from build123d import *

# Parameters (mm, degrees)
CROQUIS1_RX                  = 19.25
CROQUIS1_RY                  = 16.2
CROQUIS1_RX_2                = 16.25
CROQUIS1_RY_2                = 13.2
SALIENTE_EXTRUIR1_DEPTH      = 33
CORTAR_EXTRUIR1_DEPTH        = 33
SALIENTE_EXTRUIR2_DEPTH      = 30
SALIENTE_EXTRUIR2_DEPTH_BACK = 30
CROQUIS4_W                   = 5.818790363
CROQUIS4_H                   = 5
CORTAR_EXTRUIR2_DEPTH        = 36
SALIENTE_EXTRUIR4_DEPTH      = 33
SALIENTE_EXTRUIR5_DEPTH      = 50
CORTAR_EXTRUIR3_DEPTH        = 50
CORTAR_EXTRUIR4_START        = -17.5
CORTAR_EXTRUIR4_DEPTH        = 17.5
CORTAR_EXTRUIR5_START        = -17.5
CORTAR_EXTRUIR5_DEPTH        = 17.5
CROQUIS11_R                  = 4.25
CORTAR_EXTRUIR6_DEPTH        = 4


with BuildPart() as part:
    # Croquis1 → Saliente-Extruir1 (new body)
    with BuildSketch(Plane(origin=(0, 0, 0), x_dir=(1, 0, 0), z_dir=(0, 1, 0))):
        with Locations(Location((0, 0), (0, 0, -90))):
            Ellipse(CROQUIS1_RX, CROQUIS1_RY)
        with Locations(Location((0, 0), (0, 0, -90))):
            Ellipse(CROQUIS1_RX_2, CROQUIS1_RY_2, mode=Mode.SUBTRACT)
    extrude(amount=SALIENTE_EXTRUIR1_DEPTH)

    # Croquis2 → Cortar-Extruir1 (cut)
    with BuildSketch(Plane(origin=(0, 33, 0), x_dir=(1, 0, 0), z_dir=(0, 1, 0))):
        Polygon((0, 0), (-7.647156017, 13.245262755), (-17.669144049, 13.245262755), (-24.728519105, -10.297452091), (-13.467362336, -13.245262755), (-7.647156017, -13.245262755), align=None)
    extrude(amount=-CORTAR_EXTRUIR1_DEPTH, mode=Mode.SUBTRACT)



with BuildPart() as body_2:
    # Croquis3 → Saliente-Extruir2 (new, two sides: drawn at the far end of the back side and taken through both)
    with BuildSketch(Plane.XY.offset(-SALIENTE_EXTRUIR2_DEPTH_BACK)):
        Polygon((16.2, 0), (22.018790363, 33), (16.2, 33), align=None)
    extrude(amount=SALIENTE_EXTRUIR2_DEPTH + SALIENTE_EXTRUIR2_DEPTH_BACK)

    # Croquis4 → Cortar-Extruir2 (cut)
    with BuildSketch(Plane(origin=(0, 33, 0), x_dir=(1, 0, 0), z_dir=(0, 1, 0))):
        with Locations((19.109395181, 27.5)):
            Rectangle(CROQUIS4_W, CROQUIS4_H)
        with Locations((19.109395181, -27.5)):
            Rectangle(CROQUIS4_W, CROQUIS4_H)
    extrude(amount=-CORTAR_EXTRUIR2_DEPTH, mode=Mode.SUBTRACT)


with BuildPart() as part_1:
    add(part.part)

    add(body_2.part)  # Saliente-Extruir4 merges body 2
    # Croquis5 → Saliente-Extruir4 (add)
    with BuildSketch(Plane(origin=(0, 33, 0), x_dir=(1, 0, 0), z_dir=(0, 1, 0))):
        Polygon((17.818457755, 0), (17.818457755, 7.5), (13.626292681, 7.5), (13.626292681, -7.5), (17.818457755, -7.5), align=None)
    extrude(amount=-SALIENTE_EXTRUIR4_DEPTH)

    # Croquis6 → Saliente-Extruir5 (add)
    with BuildSketch(Plane(origin=(0, 0, -25), x_dir=(-1, 0, 0), z_dir=(0, 0, -1))):
        Polygon((-22.018790363, 33), (-16.2, 0), (-19.345508023, -0.554637933), (-25.072873954, 31.926868346), (-25.262096019, 33), align=None)
    extrude(amount=-SALIENTE_EXTRUIR5_DEPTH)

    # Croquis7 → Cortar-Extruir3 (cut)
    with BuildSketch(Plane.XY.offset(25)):
        Polygon((16.2, 0), (19.443305655, 0), (19.345508023, -0.554637933), align=None)
    extrude(amount=-CORTAR_EXTRUIR3_DEPTH, mode=Mode.SUBTRACT)

    # Croquis8 → Cortar-Extruir4 (cut)
    with BuildSketch(Plane.XY.offset(25).offset(CORTAR_EXTRUIR4_START)):
        Polygon((16.2, 0), (22.018790363, 33), (16.2, 33), align=None)
    extrude(amount=CORTAR_EXTRUIR4_DEPTH, mode=Mode.SUBTRACT)

    # Croquis9 → Cortar-Extruir5 (cut)
    with BuildSketch(Plane(origin=(0, 0, -25), x_dir=(-1, 0, 0), z_dir=(0, 0, -1)).offset(CORTAR_EXTRUIR5_START)):
        Polygon((-16.2, 0), (-22.018790363, 33), (-16.2, 33), align=None)
    extrude(amount=CORTAR_EXTRUIR5_DEPTH, mode=Mode.SUBTRACT)

    # Croquis11 → Cortar-Extruir6 (cut)
    with BuildSketch(Plane(origin=(18.857018252, -3.325001094, 0), x_dir=(0, 0, -1), z_dir=(0.984807753012208, -0.17364817766693103, 0))):
        with Locations(Location((-15, 20.130372787, 0), (0, 0, 90))):
            Circle(CROQUIS11_R)
        with Locations(Location((15, 20.130372787, 0), (0, 0, 90))):
            Circle(CROQUIS11_R)
    extrude(amount=-CORTAR_EXTRUIR6_DEPTH, mode=Mode.SUBTRACT)


solid = part_1.part
For this review, take the finished solid that the model builds, in its own axes (mm). A direction names the side the tool comes from. Round coordinates to 2 decimals unless told otherwise and drop trailing zeros. Use one line per item in the form item = value.
Item 1: Tool access review of faces 1 (the flat face through (18.42, 12.6, -16.13)), 2 (the cylindrical face through (20.64, 15.87, -19.15)), 3 (the flat face through (-10, 17, 13.245)), 4 (the flat face through (18, 20, 7.5)), 5 (the flat face through (14, 0, -2)): name each direction out of +Z, -Z, +X, -X, +Y, -Y from which nothing blocks a thin tool from reaching the whole face with its end or side.
Answers:
face_1 = -Z, +Y
face_2 = none
face_3 = -X, +Y, -Y
face_4 = +Z, +Y
face_5 = +Z, -Z, +X, -X, -Y
Item 2: Clearance check with flat-ended pins moving along their axes: P1, Ø1, axis at x = 10, z = -8, coming from the +Y side; P2, Ø8, axis at x = 18, y = 14, coming from the -Z side; P3, Ø4.5, axis at x = -10, y = 9, coming from the -Z side; P4, Ø3, axis at x = 5, y = 22, coming from the +Z side. State where each tip first meets the part, or that it passes through.
Answers:
P1 = through
P2 = -25
P3 = -16.9
P4 = 18.8
Item 3: Consider section A-A on y = 18. State how many separate pieces and enclosed holes the cut face has, then the cut area to 3 significant figures.
Answers:
separate_pieces = 3
enclosed_holes = 0
area = 383 mm^2
Item 4: Mouldability with a two-part tool opening along X and no side actions: class faces 6 (the flat face through (18, 20, -7.5)), 7 (the flat face through (-10, 17, -13.245)) as +X half, -X half, draft (parallel to the pull), parting line (faces both ways), or undercut.
Answers:
face_6 = undercut
face_7 = draft
Item 5: For line 1 (X direction, y = 23, z = -14.5); line 2 (Z direction, x = 11, y = 20.5); line 3 (Z direction, x = 3.5, y = 31), list the stretches that pass through material, from the lowest coordinate up.
Answers:
line_1 = -10.66 to -5.96, 5.96 to 10.66, 20.26 to 23.5
line_2 = -14.13 to -8.98, 8.98 to 14.13
line_3 = -18.8 to -15.67, 15.67 to 18.8
